Geometry: final body of the model. Coordinates: model frame, mm. A direction names the side the tool comes from. Round coordinates to 2 decimals unless told otherwise and drop trailing zeros. Write each loop counter-clockwise with the first axis right and the second up, starting at its lowest first coordinate (ties: lowest second). Pieces come first, ordered by that corner, then holes. Notation, with made-up numbers: (50, 65) -> (68, 65) arc R17 ccw to (68, 86) -> close; hole circle Ø11 at (-31.75, 63.25). An arc over 180 degrees is marked (long way). Use one line per item in the form item = value. Start each with the question number.
1. Reachability of faces 1 (the face through (-3, 6.35, 177)), 2 (the face through (-6.35, 9, 100)), 3 (the face through (-3, 6.35, 13)) from +Z, -Z, +X, -X, +Y, -Y: full face, straight path, thin tool, end or side. Return the list, or none.
2. Pin query (flat end, axial travel): pin 1 Ø3 at (x, y) = (-3.5, 4) entering from +Z; pin 2 Ø3 at (y, z) = (10.5, 50.5) entering from +X; pin 3 Ø1.9 at (x, z) = (-4, 184.5) entering from -Y. Return the tip coordinate at first contact, or that it passes through.
3. Line query: L1, parallel to Z at x = -0.25, y = 4.25; L2, parallel to Y at x = -3.5, z = 163.5; L3, parallel to Y at x = -5, z = 19. Output: solid intervals per line, ascending.
4. Cut plane B-B, the plane y = 3.5. Return the cut outline in (x, z).
5. Cut plane C-C, the plane z = 45. Return the cut outline in (x, y), plus the area to 3 significant figures.
6. Cut plane A-A, the plane x = -2. Return the cut outline in (y, z).
```python
from build123d import *

# Parameters (mm, degrees)
SKETCH1_W           = 6.35
SKETCH1_H           = 19.05
BOSS_EXTRUDE1_DEPTH = 203.2
SKETCH2_W           = 50.8
SKETCH2_H           = 6.35
CUT_EXTRUDE1_DEPTH  = 203.2
CUT_EXTRUDE2_DEPTH  = 203.2


with BuildPart() as part:
    # Sketch1 → Boss-Extrude1 (new body)
    with BuildSketch(Plane.XY):
        with Locations((-3.175, 9.525)):
            Rectangle(SKETCH1_W, SKETCH1_H)
    extrude(amount=BOSS_EXTRUDE1_DEPTH)

    # Sketch2 → Cut-Extrude1 (cut)
    with BuildSketch(Plane.ZY.offset(6.35)):
        with Locations((177.8, 3.175)):
            Rectangle(SKETCH2_W, SKETCH2_H)
    extrude(amount=-CUT_EXTRUDE1_DEPTH, mode=Mode.SUBTRACT)

    # Sketch3 → Cut-Extrude2 (cut)
    with BuildSketch(Plane.ZY.offset(6.35)):
        Polygon((0, 6.35), (25.4, 6.35), (50.8, 19.05), (0, 19.05), align=None)
    extrude(amount=-CUT_EXTRUDE2_DEPTH, mode=Mode.SUBTRACT)


solid = part.part
```
Outcome:
q1.face_1 = +Z, +X, -X, -Y
q1.face_2 = +Z, -Z, -X, +Y, -Y
q1.face_3 = -Z, +X, -X, +Y
q2.pin_1 = 152.4
q2.pin_2 = 0
q2.pin_3 = 6.35
q3.L1 = 0 to 152.4
q3.L2 = 6.35 to 19.05
q3.L3 = 0 to 6.35
q4.outline = (-6.35, 0) -> (0, 0) -> (0, 152.4) -> (-6.35, 152.4) -> close
q5.outline = (-6.35, 0) -> (0, 0) -> (0, 16.15) -> (-6.35, 16.15) -> close
q5.area = 103 mm^2
q6.outline = (0, 0) -> (6.35, 0) -> (6.35, 25.4) -> (19.05, 50.8) -> (19.05, 203.2) -> (6.35, 203.2) -> (6.35, 152.4) -> (0, 152.4) -> close
